Model file for the job. Use its own axes, mm. Coordinates: 2 decimals unless noted, no trailing zeros. Loops run counter-clockwise (first coordinate to the right, second up) from the corner with the lowest first, then second, coordinate; pieces in that order, holes last. Notation, with made-up numbers: (-11, -21.75) -> (42, -21.75) arc R32 ccw to (42, 8.25) -> close; hole circle Ø3 at (84.25, -31). An arc over 180 degrees is marked (long way). Use one line per item in the form item = value.
```python
from build123d import *

# Parameters (mm, degrees)
BOSS_EXTRU_1_START = 35
BOSS_EXTRU_1_DEPTH = 20


with BuildPart() as part:
    # Esquisse1 → Boss.-Extru.1 (new body)
    with BuildSketch(Plane(origin=(-30.798605227, 19.249128267, 0), x_dir=(0, 0, 1), z_dir=(-0.8479983040028684, 0.5299989400067315, 0)).offset(BOSS_EXTRU_1_START)):
        with BuildLine():
            ThreePointArc((-145, -8.476131376), (-147.928932188, -1.405063564), (-155, 1.523868624))
            Line((-155, 1.523868624), (-155, -18.476131376))
            ThreePointArc((-155, -18.476131376), (-147.928932188, -15.547199188), (-145, -8.476131376))
        make_face()
        with BuildLine():
            Line((-155, -18.476131376), (-155, 1.523868624))
            ThreePointArc((-155, 1.523868624), (-165, -8.476131376), (-155, -18.476131376))
        make_face()
        with BuildLine():
            Line((-114.7986167, 1.523868624), (-155, 1.523868624))
            ThreePointArc((-155, 1.523868624), (-147.928932188, -1.405063564), (-145, -8.476131376))
            ThreePointArc((-145, -8.476131376), (-147.928932188, -15.547199188), (-155, -18.476131376))
            Line((-155, -18.476131376), (-114.7986167, -18.476131376))
            ThreePointArc((-114.7986167, -18.476131376), (-124.7986167, -8.476131376), (-114.7986167, 1.523868624))
        make_face()
        with BuildLine():
            ThreePointArc((-104.7986167, -8.476131376), (-107.727548888, -1.405063564), (-114.7986167, 1.523868624))
            Line((-114.7986167, 1.523868624), (-114.7986167, -18.476131376))
            ThreePointArc((-114.7986167, -18.476131376), (-107.727548888, -15.547199188), (-104.7986167, -8.476131376))
        make_face()
        with BuildLine():
            Line((-114.7986167, -18.476131376), (-114.7986167, 1.523868624))
            ThreePointArc((-114.7986167, 1.523868624), (-124.7986167, -8.476131376), (-114.7986167, -18.476131376))
        make_face()
    extrude(amount=-BOSS_EXTRU_1_DEPTH)


solid = part.part
```
Q1. Pin check, flat tips, straight feed: pin 1 Ø8 at (x, y) = (-51, 28) entering from +Z; pin 2 Ø10 at (y, z) = (35.5, -111) entering from +X; pin 3 Ø12 at (x, y) = (-59.5, 23) entering from -Z; pin 4 Ø5 at (y, z) = (18, -112.5) entering from -X. Stop position of each tip, or through.
Result:
pin_1 = -104.87
pin_2 = -46.8
pin_3 = -165
pin_4 = -67.27
Q2. Wall check: line 1 along Y through (x, z) = (-53.75, -149); line 2 along X through (y, z) = (23, -162); line 3 along Y through (x, z) = (-44, -133.5). Give the ranges that are in metal, low to high.
Result:
line_1 = 11.81 to 35.39
line_2 = -66.27 to -46.14
line_3 = 26.43 to 29.3
Q3. Band-saw the part on A-A, the plane z = -138. Write the cut outline in (x, y).
Result:
outline = (-70.27, 22.13) -> (-53.31, 11.53) -> (-42.71, 28.49) -> (-59.67, 39.09) -> close
Q4. Band-saw the part on B-B, the plane z = -111.5. Write the cut outline in (x, y), and give its area (3 significant figures).
Result:
outline = (-69.97, 22.61) -> (-53.01, 12.01) -> (-43.01, 28.02) -> (-59.97, 38.62) -> close
area = 378 mm2
